Work out the finished part from the listing and answer in its coordinate system (mm). Round coordinates to 2 decimals unless told otherwise and drop trailing zeros. Order: outer loops, then holes, each group sorted by start corner. A loop starts at its lowest first (then second) coordinate and runs counter-clockwise, first axis right, second up. Notation, with made-up numbers: (34, 0.5) - (47, 0.5) arc R9 cw to (47, 14.5) - close; hole circle Ø7 at (32.5, 72.5). An arc over 180 degrees is marked (long way). Answer in a Markdown table with one row per item.
from build123d import *

# Parameters (mm, degrees)
SKETCH_1_R               = 50
SKETCH_1_R_2             = 3
SKETCH_1_R_3             = 2
EXTRUDE_1_DEPTH          = 20
SKETCH_3_R               = 82.232653787
CUT_EXTRUDE_1_DEPTH      = 10
EXTRUDE_START            = 9.3
SKETCH_4_R               = 50
EXTRUDE_2_DEPTH          = 9.3
CUT_EXTRUDE_START        = -52
SKETCH_5_R               = 3
SKETCH_5_R_2             = 2
CUT_EXTRUDE_2_DEPTH      = 52
PATTERN_CIRCULAR_1_COUNT = 6


with BuildPart() as part:
    # 草图1 → 凸台-拉伸1 (new body)
    with BuildSketch(Plane.XY):
        Circle(SKETCH_1_R)
        with Locations((-35, 0)):
            Circle(SKETCH_1_R_2, mode=Mode.SUBTRACT)
        with Locations((-17.5, 30.310889132)):
            Circle(SKETCH_1_R_2, mode=Mode.SUBTRACT)
        with Locations((17.5, 30.310889132)):
            Circle(SKETCH_1_R_2, mode=Mode.SUBTRACT)
        with Locations((35, 0)):
            Circle(SKETCH_1_R_2, mode=Mode.SUBTRACT)
        with Locations((17.5, -30.310889132)):
            Circle(SKETCH_1_R_2, mode=Mode.SUBTRACT)
        with Locations((-17.5, -30.310889132)):
            Circle(SKETCH_1_R_2, mode=Mode.SUBTRACT)
        with Locations((-23, 0)):
            Circle(SKETCH_1_R_3, mode=Mode.SUBTRACT)
        with Locations((-11.5, 19.918584287)):
            Circle(SKETCH_1_R_3, mode=Mode.SUBTRACT)
        with Locations((11.5, 19.918584287)):
            Circle(SKETCH_1_R_3, mode=Mode.SUBTRACT)
        with Locations((23, 0)):
            Circle(SKETCH_1_R_3, mode=Mode.SUBTRACT)
        with Locations((11.5, -19.918584287)):
            Circle(SKETCH_1_R_3, mode=Mode.SUBTRACT)
        with Locations((-11.5, -19.918584287)):
            Circle(SKETCH_1_R_3, mode=Mode.SUBTRACT)
    extrude(amount=EXTRUDE_1_DEPTH)

    # 草图3 → 切除-拉伸1 (cut)
    with BuildSketch(Plane.XY.offset(20)):
        Circle(SKETCH_3_R)
    extrude(amount=-CUT_EXTRUDE_1_DEPTH, mode=Mode.SUBTRACT)

    # 草图4 → 凸台-拉伸2 (add)
    with BuildSketch(Plane(origin=(0, 0, 0), x_dir=(-1, 0, 0), z_dir=(0, 0, -1)).offset(EXTRUDE_START)):
        Circle(SKETCH_4_R)
    extrude(amount=-EXTRUDE_2_DEPTH)

    # 草图5 → 切除-拉伸2 (cut)
    with BuildSketch(Plane.XY.offset(10).offset(CUT_EXTRUDE_START)):
        with Locations(Location((-35, 0, 0), (0, 0, 180))):
            Circle(SKETCH_5_R)
        with Locations(Location((-23, 0, 0), (0, 0, 180))):
            Circle(SKETCH_5_R_2)
    cut_extrude_2 = extrude(amount=CUT_EXTRUDE_2_DEPTH, mode=Mode.SUBTRACT)

    # 阵列(圆周)1: 切除-拉伸2 ×6 about axis
    pattern_circular_1_axis = Axis((0, 0, 20), (0, 0, -1))
    for i in range(1, PATTERN_CIRCULAR_1_COUNT):
        add(cut_extrude_2.rotate(pattern_circular_1_axis, i * 360 / PATTERN_CIRCULAR_1_COUNT), mode=Mode.SUBTRACT)


solid = part.part
1) Find section D-D, the plane y = -40. Give the vertices of the cut face in (x, z).
Filled in:
| item | result |
|---|---|
| outline | (-30, -9.3) - (30, -9.3) - (30, 10) - (-30, 10) - close |
2) Find the intervals of material crossed by probe 1 along Y at (x, z) = (17.5, 4); probe 2 along X at (y, z) = (-31, -3.25); probe 3 along Y at (x, z) = (11.5, 5.75), in increasing order. Write a range as from..to.
Filled in:
| item | result |
|---|---|
| probe 1 | y = -46.84..-33.31, -27.31..27.31, 33.31..46.84 |
| probe 2 | x = -39.23..-20.42, -14.58..14.58, 20.42..39.23 |
| probe 3 | y = -48.66..-21.92, -17.92..17.92, 21.92..48.66 |
3) Find section A-A, the plane z = 3. Give the number of separate pieces and of enclosed holes in the cut face, then the cut area to 3 significant figures.
Filled in:
| item | result |
|---|---|
| separate pieces | 1 |
| enclosed holes | 12 |
| area | 7,610 mm^2 |
4) Find section C-C, the plane x = -17.5. Give the vertices of the cut face in (y, z), then the cut area to 3 significant figures.
Filled in:
| item | result |
|---|---|
| outline | (-46.84, -9.3) - (-33.31, -9.3) - (-33.31, 10) - (-46.84, 10) - close; (-27.31, -9.3) - (27.31, -9.3) - (27.31, 10) - (-27.31, 10) - close; (33.31, -9.3) - (46.84, -9.3) - (46.84, 10) - (33.31, 10) - close |
| area | 1,580 mm^2 |
5) Each of these flat-tipped pins is pushed along its axis until it touches: pin 1 (8 mm diameter, centred on x = 21, z = 1, fed in from -Y); pin 2 (5 mm diameter, centred on x = 27.5, z = -6, fed in from -Y); pin 3 (6 mm diameter, centred on y = 9.5, z = -5.5, fed in from +X). Where does it stop, or does it pass through?
Filled in:
| item | result |
|---|---|
| pin 1 | stops at y = -47.02 |
| pin 2 | stops at y = -43.3 |
| pin 3 | stops at x = 49.58 |
6) Find section B-B, the plane x = 36. Give the vertices of the cut face in (y, z).
Filled in:
| item | result |
|---|---|
| outline | (-34.7, -9.3) - (-2.83, -9.3) - (-2.83, 10) - (-34.7, 10) - close; (2.83, -9.3) - (34.7, -9.3) - (34.7, 10) - (2.83, 10) - close |
